Check sheet for the modelled part. Datum: model origin and axes. Units: mm. A direction names the side the tool comes from. Coordinates: 2 decimals unless noted, no trailing zeros. Loops run counter-clockwise (first coordinate to the right, second up) from the corner with the lowest first, then second, coordinate; pieces in that order, holes last. Notation, with made-up numbers: M 15.25,-4 L 71.25,-4 A20 ccw 71.25,25 Z; hole C -35.5,19 d8. An arc over 180 degrees is marked long. Write each question's results on one line, items separated by ' | '. Start each with the question number.
from build123d import *

# Parameters (mm, degrees)
F4_T = -2.54


with BuildPart() as f3:
    # F0 (on Top) → F3 section 0
    with BuildSketch(Plane.XY, mode=Mode.PRIVATE) as f3_s0:
        Polygon((-30.354286, 41.401532), (-50.739026, 7.811583), (-41.401532, -30.354286), (-7.811583, -50.739026), (30.354286, -41.401532), (50.739026, -7.811583), (41.401532, 30.354286), (7.811583, 50.739026), align=None)
    loft([f3_s0.sketch, Vertex(0, 0, 76.2)])

    # F4
    f4_openings = [f3.faces().sort_by_distance(p)[0] for p in [
        (0, 0, 0),
    ]]
    offset(amount=F4_T, openings=f4_openings)


solid = f3.part
1) Section check A-A (z = 27). Enter the section's corners in (x, y).
2) Gauge pin test, flat ends, axial feed: P1, Ø3, axis at y = 10, z = 58.5, coming from the -X side; P2, Ø1, axis at x = -14, z = 49, coming from the -Y side; P3, Ø2, axis at x = 22, y = -36.5, coming from the +Z side. Record the tip position at first contact, or that the pin passes through.
3) Thickness scan on probe 1 along Y at (x, z) = (-17, 8.5); probe 2 along X at (y, z) = (4, 18); probe 3 along Y at (x, z) = (-18, 27). Record the ranges inside material, lowest first.
4) Section check C-C (x = 17.5). Enter the section's corners in (y, z), then the cut area to 3 significant figures.
5) Section check B-B (y = -21). Enter the section's corners in (x, z), then the cut area to 3 significant figures.
6) Release check for a two-part mould opening along X. For faces 1 (the flat face through (-15.1, -24.35, 30.17)), 2 (the flat face through (-14.148, -22.816, 28.264)), 3 (the flat face through (6.542, -27.897, 30.167)) record: +X half, -X half, draft (parallel to the pull), parting line (faces both ways), or undercut.
7) Set-up check for faces 4 (the flat face through (-13, 43, 0)), 5 (the flat face through (6.13, -26.14, 28.26)): record each of +Z, -Z, +X, -X, +Y, -Y from which the full face is reachable in a straight line by a thin tool's end or side.
8) Section check D-D (z = 5). Enter the section's corners in (x, y), then the cut area to 3 significant figures.
Return value:
1) outline: M -32.76,5.04 L -26.73,-19.6 L -5.04,-32.76 L 19.6,-26.73 L 32.76,-5.04 L 26.73,19.6 L 5.04,32.76 L -19.6,26.73 Z; hole M -29.56,4.55 L -24.12,-17.68 L -4.55,-29.56 L 17.68,-24.12 L 29.56,-4.55 L 24.12,17.68 L 4.55,29.56 L -17.68,24.12 Z
2) P1: stops at x = -8.24 | P2: stops at y = -11.78 | P3: stops at z = 12.45
3) probe 1: y = -38.97 to -35.47, 36.14 to 39.22 | probe 2: x = -38.27 to -35.19, 33.24 to 36.32 | probe 3: y = -24.9 to -21.4, 23.6 to 27.12
4) outline: M -44.55,0 L -41.47,0 L -23.87,27.46 L -2.69,45.11 L 12.83,39.18 L 41.36,0 L 44.86,0 L 12.83,43.99 L -2.69,49.92 L -23.87,32.27 Z | area: 414 mm2
5) outline: M -43.69,0 L -40.61,0 L -28.64,18.68 L -3.23,39.86 L 15.4,32.74 L 39.24,0 L 42.74,0 L 15.4,37.55 L -3.23,44.66 L -28.64,23.48 Z | area: 400 mm2
6) face 1: -X half | face 2: undercut | face 3: +X half
7) face 4: -Z, +X, -X, +Y, -Y | face 5: -Z
8) outline: M -47.41,7.3 L -38.68,-28.36 L -7.3,-47.41 L 28.36,-38.68 L 47.41,-7.3 L 38.68,28.36 L 7.3,47.41 L -28.36,38.68 Z; hole M -44.21,6.81 L -36.07,-26.45 L -6.81,-44.21 L 26.45,-36.07 L 44.21,-6.81 L 36.07,26.45 L 6.81,44.21 L -26.45,36.07 Z | area: 849 mm2
